```python
from build123d import *

# Parameters (mm, degrees)
SKETCH_1_W             = 35
SKETCH_1_H             = 15
EXTRUDE_1_DEPTH        = 2.4
FILLET_1_R             = 0.5
SKETCH_2_W             = 35
SKETCH_2_H             = 11
EXTRUDE_2_DEPTH        = 2.6
SKETCH_3_W             = 3.5
SKETCH_3_H             = 2
EXTRUDE_3_DEPTH        = 2.6
CUT_EXTRUDE_1_DEPTH    = 15
CUT_EXTRUDE_2_DEPTH    = 5
CUT_EXTRUDE_3_DEPTH    = 2.4
EXTRUDE_4_DEPTH        = 2.4
CUT_EXTRUDE_4_DEPTH    = 2.4
FILLET_2_R             = 0.5
FILLET_2_OF_MIRROR_2_R = 0.5
SKETCH_17_W            = 3
SKETCH_17_H            = 5
CUT_EXTRUDE_5_DEPTH    = 15
SKETCH_18_W            = 3
SKETCH_18_H            = 6
CUT_EXTRUDE_6_DEPTH    = 5


with BuildPart() as part:
    # 草图1 → 凸台-拉伸1 (new body)
    with BuildSketch(Plane(origin=(0, 0, 0), x_dir=(1, 0, 0), z_dir=(0, 1, 0))):
        with Locations((17.5, 7.5)):
            Rectangle(SKETCH_1_W, SKETCH_1_H)
    extrude(amount=EXTRUDE_1_DEPTH)

    # 圆角1
    fillet_1_edges = [part.edges().sort_by_distance(p)[0] for p in [
        (17.5, 2.4, -15),
        (17.5, 2.4, 0),
    ]]
    fillet(fillet_1_edges, radius=FILLET_1_R)

    # 草图2 → 凸台-拉伸2 (add)
    with BuildSketch(Plane.XZ):
        with Locations((17.5, -7.5)):
            Rectangle(SKETCH_2_W, SKETCH_2_H)
    extrude(amount=EXTRUDE_2_DEPTH)

    # 草图3 → 凸台-拉伸3 (add)
    with BuildSketch(Plane.XZ):
        with Locations((33.25, -1)):
            Rectangle(SKETCH_3_W, SKETCH_3_H)
    extrude_3 = extrude(amount=EXTRUDE_3_DEPTH)

    # 镜向1: 凸台-拉伸3 across plane
    add(extrude_3.mirror(Plane(origin=(0, 0, -7.5), x_dir=(1, 0, 0), z_dir=(0, 0, -1))))

    # 草图4 → 切除-拉伸1 (cut)
    with BuildSketch(Plane(origin=(0, 0, -15), x_dir=(-1, 0, 0), z_dir=(0, 0, -1))):
        Polygon((-35, -1.1), (-33, 0.9), (-33, 2.4), (-35, 2.4), align=None)
    extrude(amount=-CUT_EXTRUDE_1_DEPTH, mode=Mode.SUBTRACT)

    # 草图6 → 切除-拉伸2 (cut)
    with BuildSketch(Plane(origin=(0, 2.4, 0), x_dir=(1, 0, 0), z_dir=(0, 1, 0))):
        with BuildLine():
            Line((12, 15), (27, 15))
            Line((27, 15), (27, 14))
            ThreePointArc((27, 14), (25.828427125, 11.171572875), (23, 10))
            Line((23, 10), (12, 10))
            Line((12, 10), (12, 15))
        make_face()
    cut_extrude_2 = extrude(amount=-CUT_EXTRUDE_2_DEPTH, mode=Mode.SUBTRACT)

    # 扫描4: sweep along a path in 草图13
    with BuildLine(Plane(origin=(0, 2.4, 0), x_dir=(1, 0, 0), z_dir=(0, 1, 0))) as sweep_4_path:
        Line((12, 14.5), (22.3, 14.5))
        ThreePointArc((22.3, 14.5), (23.148528137, 14.851471863), (23.5, 15.7))
        Line((23.5, 15.7), (23.5, 16))
    # 草图10 → 扫描4 (sweep)
    with BuildSketch(Plane(origin=(0, 0, -16), x_dir=(-1, 0, 0), z_dir=(0, 0, -1))):
        with BuildLine():
            Line((-25, 2.4), (-23.5, 2.4))
            ThreePointArc((-23.5, 2.4), (-23.146446609, 2.253553391), (-23, 1.9))
            Line((-23, 1.9), (-23, 0))
            Line((-23, 0), (-25, 0))
            Line((-25, 0), (-25, 2.4))
        make_face()
    sweep_4 = sweep(path=sweep_4_path.line)

    # 草图14 → 切除-拉伸3 (cut)
    with BuildSketch(Plane.XZ):
        Polygon((22.721496019, -16), (22.721496019, -15.221496019), (23.5, -16), align=None)
        Polygon((25.109405679, -16), (25.109405679, -14.890594321), (24, -16), align=None)
    cut_extrude_3 = extrude(amount=-CUT_EXTRUDE_3_DEPTH, mode=Mode.SUBTRACT)

    # 草图15 → 凸台-拉伸4 (add)
    with BuildSketch(Plane.XZ):
        with BuildLine():
            Line((12, -10), (12, -13))
            Line((12, -13), (16, -13))
            ThreePointArc((16, -13), (14.774754878, -12.626225608), (13.5, -12.5))
            ThreePointArc((13.5, -12.5), (13.146446609, -12.353553391), (13, -12))
            Line((13, -12), (13, -11))
            ThreePointArc((13, -11), (13.146446609, -10.646446609), (13.5, -10.5))
            ThreePointArc((13.5, -10.5), (14.794008988, -10.470044942), (16, -10))
            Line((16, -10), (12, -10))
        make_face()
    extrude_4 = extrude(amount=-EXTRUDE_4_DEPTH)

    # 草图16 → 切除-拉伸4 (cut)
    with BuildSketch(Plane.XZ):
        with BuildLine():
            Line((16, -13), (22.3, -13))
            ThreePointArc((22.3, -13), (23.338390931, -13.207662889), (24.217052039, -13.798707945))
            ThreePointArc((24.217052039, -13.798707945), (20.040683481, -14.097313313), (16, -13))
        make_face()
    cut_extrude_4 = extrude(amount=-CUT_EXTRUDE_4_DEPTH, mode=Mode.SUBTRACT)

    # 圆角2
    fillet_2_edges = [part.edges().sort_by_distance(p)[0] for p in [
        (23.5, 1.2, -16),
        (24, 1.2, -16),
    ]]
    fillet(fillet_2_edges, radius=FILLET_2_R)

    # 镜向2: 切除-拉伸2, 扫描4, 切除-拉伸3, 凸台-拉伸4, 切除-拉伸4 across plane
    add(cut_extrude_2.mirror(Plane.XY.offset(-7.5)), mode=Mode.SUBTRACT)
    add(sweep_4.mirror(Plane.XY.offset(-7.5)))
    add(cut_extrude_3.mirror(Plane.XY.offset(-7.5)), mode=Mode.SUBTRACT)
    add(extrude_4.mirror(Plane.XY.offset(-7.5)))
    add(cut_extrude_4.mirror(Plane.XY.offset(-7.5)), mode=Mode.SUBTRACT)

    # 圆角2 of 镜向2
    fillet_2_of_mirror_2_edges = [part.edges().sort_by_distance(p)[0] for p in [
        (23.5, 1.2, 1),
        (24, 1.2, 1),
    ]]
    fillet(fillet_2_of_mirror_2_edges, radius=FILLET_2_OF_MIRROR_2_R)

    # 草图17 → 切除-拉伸5 (cut)
    with BuildSketch(Plane(origin=(0, 0, -15), x_dir=(-1, 0, 0), z_dir=(0, 0, -1))):
        with Locations((-1.5, -0.1)):
            Rectangle(SKETCH_17_W, SKETCH_17_H)
    extrude(amount=-CUT_EXTRUDE_5_DEPTH, mode=Mode.SUBTRACT)

    # 草图18 → 切除-拉伸6 (cut)
    with BuildSketch(Plane(origin=(0, 2.4, 0), x_dir=(1, 0, 0), z_dir=(0, 1, 0))):
        with Locations((6.5, 7.5)):
            Rectangle(SKETCH_18_W, SKETCH_18_H)
    extrude(amount=-CUT_EXTRUDE_6_DEPTH, mode=Mode.SUBTRACT)


solid = part.part
```
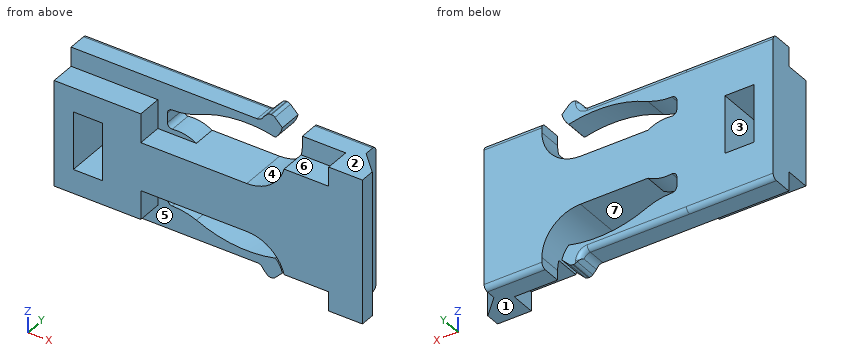
CAD build for the part. Positions are in the model's coordinates, mm. Face numbers are marked on the shaded views. A direction names the side the tool comes from. Coordinates: 2 decimals unless noted, no trailing zeros. Order: outer loops, then holes, each group sorted by start corner. A loop starts at its lowest first (then second) coordinate and runs counter-clockwise, first axis right, second up. Notation, with made-up numbers: M 13,83.25 L 69,83.25 A10 ccw 69,101.25 Z; hole C 32.5,-16 d4. An arc over 180 degrees is marked long. Write each question's results on one line, items separated by ' | '. Start each with the question number.
Q1. Flat gauge pins, fed straight in: P1, Ø3, axis at y = 1.5, z = -7.5, coming from the +X side; P2, Ø3, axis at x = 28.5, y = -2, coming from the -Z side; P3, Ø1.6, axis at y = 1.5, z = -6, coming from the +X side; P4, Ø6, axis at x = 24, z = -2.5, coming from the +Y side. Where does each tip first touch, or does it go through?
Q2. Pull direction Z, two halves, no side cores. Call the marked faces 4, 5, 6 and 7: +Z half, -Z half, draft (parallel to the pull), parting line (faces both ways), or undercut.
Q3. Cut at B-B (y = -1.4). List the corners of the cut face in (x, z).
Q4. Drill centre lines: probe 1 along Z at (x, y) = (7.5, -2.2); probe 2 along X at (y, z) = (1.15, -7.25); probe 3 along Z at (x, y) = (15, 1.7). Where is each one in solid material? Low to high. Write a range as from..to.
Q5. Which spindle directions (+Z, -Z, +X, -X, +Y, -Y) get a long thin tool onto all of the face, cutting with end or side? Do the marked faces 1, 2 and 3. Say none if no direction does.
Q6. Cut at A-A (z = -6.75). List the corners of the cut face in (x, y), then the cut area to 3 significant figures.
Q7. Cut at D-D (x = 30.5). List the corners of the cut face in (y, z).
Q8. Cut at C-C (x = 15.5). List the corners of the cut face in (y, z), then the cut area to 3 significant figures.
Found:
1) P1: x = 33.9 | P2: z = -13 | P3: x = 33.2 | P4: y = 2.4
2) face 4: undercut | face 5: draft | face 6: +Z half | face 7: undercut
3) outline: M 3,-13 L 12,-13 L 12,-10 L 23,-10 A4 cw 26.87,-13 L 31.5,-13 L 31.5,-15 L 35,-15 L 35,0 L 31.5,0 L 31.5,-2 L 26.87,-2 A4 cw 23,-5 L 12,-5 L 12,-2 L 3,-2 Z; hole M 5,-10.5 L 8,-10.5 L 8,-4.5 L 5,-4.5 Z
4) probe 1: -13..-10.5, -4.5..-2 | probe 2: 3..5, 8..33 | probe 3: -15..-12.68, -10.42..-4.58, -2.32..0
5) face 1: -Z, +X, +Y, -Y | face 2: +Z, +X, +Y, -Y | face 3: +Y, -Y
6) outline: M 3,-2.6 L 5,-2.6 L 5,2.4 L 3,2.4 Z; M 8,-2.6 L 35,-2.6 L 35,-1.1 L 33,0.9 L 33,2.4 L 8,2.4 Z | area: 140 mm²
7) outline: M -2.6,-13 L 0,-13 L 0,-15 L 1.9,-15 A0.5 ccw 2.4,-14.5 L 2.4,-0.5 A0.5 ccw 1.9,0 L 0,0 L 0,-2 L -2.6,-2 Z
8) outline: M -2.6,-10 L 0,-10 L 0,-10.25 L 2.4,-10.25 L 2.4,-4.75 L 0,-4.75 L 0,-5 L -2.6,-5 Z; M 0,-15 L 1.9,-15 A0.5 ccw 2.4,-14.5 L 2.4,-12.82 L 0,-12.82 Z; M 0,-2.18 L 2.4,-2.18 L 2.4,-0.5 A0.5 ccw 1.9,0 L 0,0 Z | area: 36.6 mm²
